Read the model definition and answer for the solid it produces. Units are mm, in the model's axes. Coordinates: 2 decimals unless noted, no trailing zeros. Write each loop counter-clockwise with the first axis right and the second up, starting at its lowest first coordinate (ties: lowest second). Pieces come first, ordered by that corner, then holes.
from build123d import *

# Parameters (mm, degrees)
SKETCH1_W               = 815
SKETCH1_H               = 222
BOSS_EXTRUDE1_DEPTH     = 10
CHAMFER1_SIZE           = 135
F_1_4_CLEARANCE_HOLE1_D = 6.7564


with BuildPart() as part:
    # Sketch1 → Boss-Extrude1 (new body)
    with BuildSketch(Plane(origin=(0, 0, 0), x_dir=(0, 0, -1), z_dir=(1, 0, 0))):
        with Locations((407.5, 111)):
            Rectangle(SKETCH1_W, SKETCH1_H)
    extrude(amount=BOSS_EXTRUDE1_DEPTH)

    # Chamfer1
    chamfer1_edges = [part.edges().sort_by_distance(p)[0] for p in [
        (5, 222, 0),
        (5, 222, -815),
    ]]
    chamfer(chamfer1_edges, length=CHAMFER1_SIZE)

    # 1/4 Clearance Hole1 (through all)
    with Locations(Plane(origin=(10, 0, 0), x_dir=(0, 0, -1), z_dir=(1, 0, 0))):
        with Locations((482.5, 65), (332.5, 65)):
            Hole(F_1_4_CLEARANCE_HOLE1_D / 2)


solid = part.part
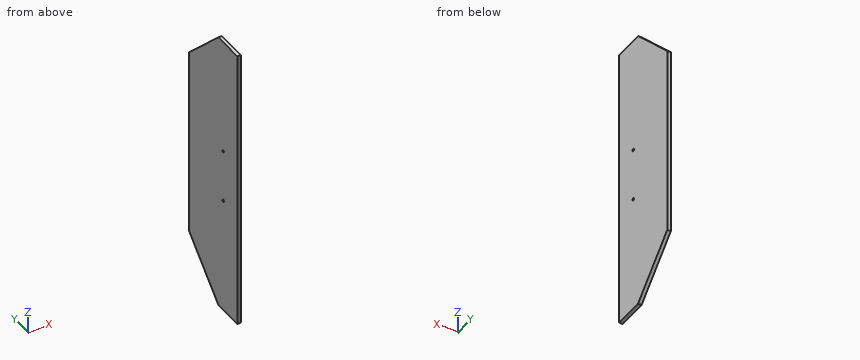
Item 1: The part is cut by section C-C (z = -68.5). Give the vertices of the cut face in (x, y).
Item 2: The part is cut by section A-A (x = 6.25). Give the vertices of the cut face in (y, z).
Item 3: Find the intervals of material crossed by probe 1 along Z at (x, y) = (7.5, 64); probe 2 along Y at (x, z) = (5.25, -332.5); probe 3 along Z at (x, y) = (1, 174), in increasing order.
Item 4: Given pin 1 (5 mm diameter, centred on x = 4, y = 118.5, fed in from -Z); pin 2 (4 mm diameter, centred on y = 65, z = -332.5, fed in from -X); pin 3 (3 mm diameter, centred on x = 7.5, y = 177, fed in from +Z), each flat-ended and moving along its own axis, determine where each tip first touches the part or whether it passes through.
Item 5: The part is cut by section B-B (y = 115). Give the vertices of the cut face in (x, z).
Answer:
1. outline: (0, 0) - (10, 0) - (10, 155.5) - (0, 155.5) - close
2. outline: (0, -815) - (87, -815) - (222, -680) - (222, -135) - (87, 0) - (0, 0) - close; hole circle Ø6.76 at (65, -482.5); hole circle Ø6.76 at (65, -332.5)
3. probe 1: z = -815 to -485.73, -479.27 to -335.73, -329.27 to 0
3. probe 2: y = 0 to 61.62, 68.38 to 222
3. probe 3: z = -728 to -87
4. pin 1: stops at z = -786
4. pin 2: passes through
4. pin 3: stops at z = -88.5
5. outline: (0, -787) - (10, -787) - (10, -28) - (0, -28) - close
